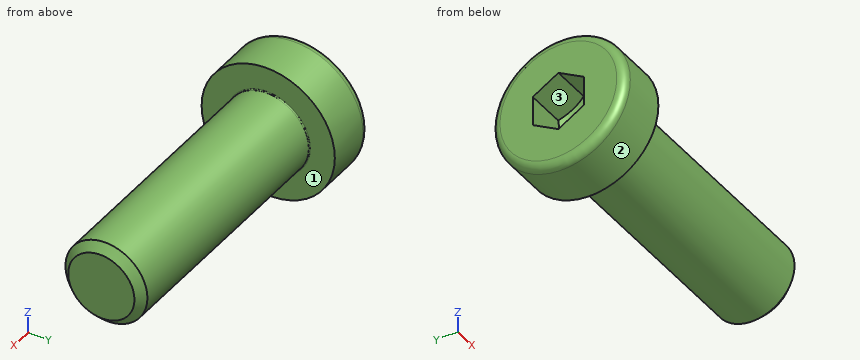
Autodesk Inventor part; units mm, degrees
ref_plane "Work Plane1" through (29, 0, 0) normal (0, -1, 0) x (1, 0, 0)
ref_plane "YZ Plane" through (0, 0, 0) normal (1, 0, 0) x (0, 1, 0)
ref_plane "XZ Plane" through (0, 0, 0) normal (0, 1, 0) x (-1, 0, 0)
sketch "Sketch1" plane through (0, 0, 0) normal (0, 0, 1) x (1, 0, 0)
  line L0 (0.4667, 0) -> (25, 0)
  line L1 (25, 0) -> (25, 4)
  line L2 (25, 4) -> (3.75, 4)
  line L3 (3.75, 4) -> (2.9831, 4)
  line L4 (2.9831, 4) -> (0, 4)
  line L5 (0, 4) -> (0, 6.5)
  line L6 (0, 6.5) -> (-5, 6.5)
  line L7 (-5, 6.5) -> (-5, 2.8868)
  line L8 (-5, 2.8868) -> (-1.2, 2.8868)
  line L9 (-1.2, 2.8868) -> (0.4667, 0)
  line L10 (-11, 0) -> (31, 0)
  line L11 (0, -1.3) -> (0, 7.8)
  line L12 (3.75, 4) -> (0, 4) construction
  dimension "d1" = 21.25
  dimension "d2" = 0.7669
  dimension "d3" = 5
  dimension "d4" = 3.8
  dimension "d5" = 60
  dimension "d6" = 8
  dimension "d7" = 8
  dimension "d8" = 5.7735
  dimension "d9" = 13
  dimension "d26" = 25
revolve "Body" add sketch "Sketch1" angle 360 about axis through (0.4667, 0, 0) along (1, 0, 0) contours L9 L11 L4 L3 L2 L1 L0 | L9 L8 L7 L6 L5 L11
sketch "Sketch2" plane through (-5, 0, 0) normal (-1, 0, 0) x (0, 0, 1)
  circle A0 centre (0, 0) radius 2.8868
  line L0 (0, -9.1) -> (0, 9.1)
  line L1 (-9.1, 0) -> (9.1, 0)
  line L2 (2.8868, 0) -> (1.4434, -2.5)
  line L3 (1.4434, -2.5) -> (-1.4434, -2.5)
  line L4 (-1.4434, -2.5) -> (-2.8868, 0)
  line L5 (-2.8868, 0) -> (-1.4434, 2.5)
  line L6 (-1.4434, 2.5) -> (1.4434, 2.5)
  line L7 (1.4434, 2.5) -> (2.8868, 0)
  point P0 (0, 0)
extrude "Slot" add sketch "Sketch2" against normal up to next contours L7 A0 | A0 L2 | L6 L0 A0 | A0 L0 L3 | L0 L6 A0 | A0 L3 L0 | L4 A0 | A0 L5
fillet "Fillet1" radius 0.8 1 edges at (-5, -6.5, 0)
thread "Thread"
chamfer "Chamfer1" distance 0.7668 distance2 0.7668 1 edges at (25, -4, 0) measured on face at (25, -0.6859, 0.8072)
ref_plane "Work Plane1" through (29, 0, 0) normal (0, -1, 0) x (1, 0, 0)
fillet "Fillet2" radius 0.1 1 edges at (0, -4, 0)
equation "\"d1\" = GEL"
equation "\"d3\" = KOH"
equation "\"d4\" = INTI"
equation "\"d6\" = GD"
equation "\"d7\" = BDM"
equation "\"d8\" = 1.1547 * SW"
equation "\"d9\" = KOD"
equation "\"d26\" = NLG"
equation "\"d30\" = R"
equation "\"d17\" = RR"
equation "\"d13\" = GEL"
equation "\"d15\" = -0.5 * SPD + 0.5 * GD"
equation "\"d16\" = GUL"
equation "\"GD\" = NND"
equation "\"NLG\" = 25"
equation "\"GEL\" = 21.25"
equation "\"KOD\" = 13"
equation "\"KOH\" = 5"
equation "\"INTI\" = 3.8"
equation "\"GAL\" = 0.61345 * PTC"
equation "\"GUL\" = 0.61345 * PTC"
equation "\"BDM\" = NND"
equation "\"SW\" = 5"
equation "\"RR\" = 0.8"
equation "\"SPD\" = NND - 1.2269 * PTC"
equation "\"R\" = 0.1"
equation "\"TOA\" = 30deg"
equation "\"GD1\" = THREADDIA - 1.2269 * PTC"
equation "\"THREADDIA\" = 8"
equation "\"FAWI\" = 45deg"
equation "\"ANG\" = 120deg"
equation "\"PTC\" = 1.25"
equation "\"NND\" = 8"
equation "\"E0\" = 1.155 * SW"
properties part number "DIN 7984 - M8 x 25" material "Steel, Mild"
Check sheet for the modelled part. Datum: model origin and axes. Units: mm. Face numbers are marked on the shaded views. A direction names the side the tool comes from. Give positions to 0.01 mm unless a question says otherwise; leave off trailing zeros. Order: outer loops, then holes, each group sorted by start corner. A loop starts at its lowest first (then second) coordinate and runs counter-clockwise, first axis right, second up. Notation, with made-up numbers: M 3.25,54 L 8.25,54 A14 cw 8.25,78 Z; hole C 26.25,24 d2. An arc over 180 degrees is marked long. Answer as CSV lines item,"result". Start each with the question number.
Item 1: Gauge pin test, flat ends, axial feed: P1, Ø5, axis at x = 11, z = 0, coming from the -Y side; P2, Ø5, axis at x = 12.5, y = -2, coming from the +Z side. Record the tip position at first contact, or that the pin passes through.
Item 2: Cross-section at A-A on x = 20. Enter the section's corners in (y, z), plus the area to 3 significant figures.
Item 3: Tool access check on the marked faces 1, 2 and 3. Record the directions out of +Z, -Z, +X, -X, +Y, -Y that give a thin tool (end or side, any length) a straight path to the whole face; none if there is none.
Item 4: Thickness scan on line 1 (X direction, y = 4.5, z = 3.5); line 2 (Z direction, x = 18.75, y = 0); line 3 (Z direction, x = -3, y = -2.25). Record the ranges inside material, lowest first. Write a range as [from, to].
Established:
1,P1,"stops at y = -4"
1,P2,"stops at z = 4"
2,outline,"C 0,0 d8"
2,area,"50.3 mm^2"
3,face 1,"+X"
3,face 2,"+X, -X"
3,face 3,"-X"
4,line 1,"x = [-5, 0]"
4,line 2,"z = [-4, 4]"
4,line 3,"z = [-6.1, -1.59], [1.59, 6.1]"
